```python
from build123d import *

# Parameters (mm, degrees)
ESBO_O1_W                                            = 300
ESBO_O1_H                                            = 19.02
ESBO_O1_R                                            = 4
RESSALTO_EXTRUS_O1_DEPTH                             = 19.02
REBAIXO_PARA_PARAFUSO_ALLEN_SEXTAVADO_DE_D           = 9
REBAIXO_PARA_PARAFUSO_ALLEN_SEXTAVADO_DE_CBORE_D     = 15
REBAIXO_PARA_PARAFUSO_ALLEN_SEXTAVADO_DE_CBORE_DEPTH = 8.6
ESBO_O5_R                                            = 4
CORTE_EXTRUS_O1_DEPTH                                = 20.02
REBAIXO_PARA_PARAFUSO_ALLEN_SEXTAVAD_2_D             = 9
REBAIXO_PARA_PARAFUSO_ALLEN_SEXTAVAD_2_CBORE_D       = 15
REBAIXO_PARA_PARAFUSO_ALLEN_SEXTAVAD_2_CBORE_DEPTH   = 8.6
ESBO_O11_R                                           = 7.5
CORTE_EXTRUS_O2_DEPTH                                = 8.6


with BuildPart() as part:
    # Esboço1 → Ressalto-extrusão1 (new body)
    with BuildSketch(Plane(origin=(0, 0, 0), x_dir=(0, 0, -1), z_dir=(1, 0, 0))):
        with Locations((0, 3.19)):
            Rectangle(ESBO_O1_W, ESBO_O1_H)
        with Locations((-50, 3.19)):
            Circle(ESBO_O1_R, mode=Mode.SUBTRACT)
        with Locations((-125, 3.19)):
            Circle(ESBO_O1_R, mode=Mode.SUBTRACT)
        with Locations((50, 3.19)):
            Circle(ESBO_O1_R, mode=Mode.SUBTRACT)
        with Locations((125, 3.19)):
            Circle(ESBO_O1_R, mode=Mode.SUBTRACT)
    extrude(amount=RESSALTO_EXTRUS_O1_DEPTH)

    # Rebaixo para parafuso Allen sextavado de (through all)
    with Locations(Plane(origin=(19.02, 3.19, 125), x_dir=(0, 0, 1), z_dir=(1, 0, 0))):
        with Locations((0, 0), (-75, 0), (-175, 0), (-250, 0)):
            CounterBoreHole(REBAIXO_PARA_PARAFUSO_ALLEN_SEXTAVADO_DE_D / 2, REBAIXO_PARA_PARAFUSO_ALLEN_SEXTAVADO_DE_CBORE_D / 2, REBAIXO_PARA_PARAFUSO_ALLEN_SEXTAVADO_DE_CBORE_DEPTH)

    # Esboço5 → Corte-extrusão1 (cut, through all)
    with BuildSketch(Plane.ZY):
        with Locations((0, 3.19)):
            Circle(ESBO_O5_R)
        with Locations((90, 3.19)):
            Circle(ESBO_O5_R)
        with Locations((-90, 3.19)):
            Circle(ESBO_O5_R)
    extrude(amount=-CORTE_EXTRUS_O1_DEPTH, mode=Mode.SUBTRACT)

    # Rebaixo para parafuso Allen sextavad 2 (through all)
    with Locations(Plane(origin=(0, 3.19, -90), x_dir=(0, 0, -1), z_dir=(-1, 0, 0))):
        with Locations((0, 0), (-180, 0)):
            CounterBoreHole(REBAIXO_PARA_PARAFUSO_ALLEN_SEXTAVAD_2_D / 2, REBAIXO_PARA_PARAFUSO_ALLEN_SEXTAVAD_2_CBORE_D / 2, REBAIXO_PARA_PARAFUSO_ALLEN_SEXTAVAD_2_CBORE_DEPTH)

    # Esboço11 → Corte-extrusão2 (cut)
    with BuildSketch(Plane.ZY):
        with Locations((0, 3.19)):
            Circle(ESBO_O11_R)
    extrude(amount=-CORTE_EXTRUS_O2_DEPTH, mode=Mode.SUBTRACT)


solid = part.part
```
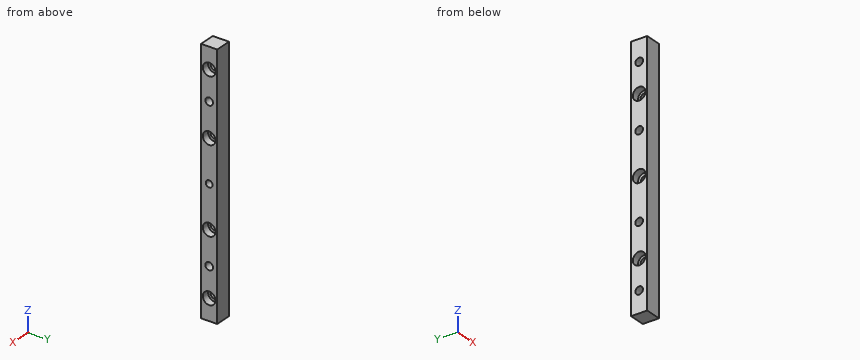
Geometry: final body of the model. Coordinates: model frame, mm. Round coordinates to 2 decimals unless told otherwise and drop trailing zeros. Write each loop counter-clockwise with the first axis right and the second up, starting at its lowest first coordinate (ties: lowest second). Pieces come first, ordered by that corner, then holes.
Item 1: Section query B-B (z = 125). Return loops of the section in (x, y).
Item 2: Section query C-C (z = 51.5). Return loops of the section in (x, y), plus the area to 3 significant figures.
Item 3: Section query A-A (x = 13). Return loops of the section in (y, z).
Item 4: Pin query (flat end, axial travel): P1, Ø10.5, axis at y = 3.19, z = -90, coming from the -X side; P2, Ø8, axis at y = 3.19, z = -125, coming from the -X side; P3, Ø4.5, axis at y = 0.5, z = 123.5, coming from the +X side. Return the tip coordinate at first contact, or that it passes through.
Item 5: Material intervals for L1, parallel to Z at x = 13, y = -2.25; L2, parallel to Z at x = 5, y = -3.75; L3, parallel to Y at x = 4.5, z = -90, sorted ascending.
Completed:
1. outline: (0, -6.32) - (19.02, -6.32) - (19.02, -4.31) - (10.42, -4.31) - (10.42, -1.31) - (0, -1.31) - close; (0, 7.69) - (10.42, 7.69) - (10.42, 10.69) - (19.02, 10.69) - (19.02, 12.7) - (0, 12.7) - close
2. outline: (0, -6.32) - (19.02, -6.32) - (19.02, -4.16) - (10.42, -4.16) - (10.42, -1.05) - (0, -1.05) - close; (0, 7.43) - (10.42, 7.43) - (10.42, 10.54) - (19.02, 10.54) - (19.02, 12.7) - (0, 12.7) - close
2. area: 147 mm2
3. outline: (-6.32, -150) - (12.7, -150) - (12.7, 150) - (-6.32, 150) - close; hole circle Ø15 at (3.19, -125); hole circle Ø15 at (3.19, -50); hole circle Ø15 at (3.19, 50); hole circle Ø15 at (3.19, 125); hole circle Ø9 at (3.19, -90); hole circle Ø9 at (3.19, 90); hole circle Ø8 at (3.19, 0)
4. P1: stops at x = 8.6
4. P2: passes through
4. P3: stops at x = 10.42
5. L1: z = -150 to -130.16, -119.84 to -55.16, -44.84 to 44.84, 55.16 to 119.84, 130.16 to 150
5. L2: z = -150 to -92.84, -87.16 to -2.84, 2.84 to 87.16, 92.84 to 150
5. L3: y = -6.32 to -4.31, 10.69 to 12.7
